Geometry check sheet. Reference: the model listing, model coordinates, mm. A direction names the side the tool comes from. Give positions to 0.01 mm unless a question says otherwise; leave off trailing zeros. Write each loop counter-clockwise with the first axis right and the second up, starting at its lowest first coordinate (ties: lowest second). Pieces come first, ordered by that corner, then holes. Notation, with made-up numbers: (-35, 31) -> (-6, 31) arc R22 cw to (-6, 60) -> close; hole circle Ø4 at (-1, 80). An arc over 180 degrees is marked (long way). One line per item, written item: value.
from build123d import *

# Parameters (mm, degrees)
V10_SHT_CANDIDATE_CARRIER16X16_START   = 54
SKETCH_2_W                             = 16
SKETCH_2_H                             = 1.6
V10_SHT_CANDIDATE_CARRIER16X16_DEPTH   = 16
V10_SHT_SENSING_PACKAGE_REARWARD_START = 60.5
SKETCH_3_W                             = 3
SKETCH_3_H                             = 1.2
V10_SHT_SENSING_PACKAGE_REARWARD_DEPTH = 3
SKETCH_4_R                             = 1.3
V10_SHT_TWO_CANDIDATE_HOLES8MM_DEPTH   = 1.6


with BuildPart() as part:
    # Sketch 2 → V10_SHT_candidate_carrier16x16 (new body)
    with BuildSketch(Plane.XY.offset(V10_SHT_CANDIDATE_CARRIER16X16_START)):
        with Locations((-122, 133.2)):
            Rectangle(SKETCH_2_W, SKETCH_2_H)
    extrude(amount=V10_SHT_CANDIDATE_CARRIER16X16_DEPTH)

    # Sketch 3 → V10_SHT_sensing_package_rearward (add)
    with BuildSketch(Plane.XY.offset(V10_SHT_SENSING_PACKAGE_REARWARD_START)):
        with Locations((-122, 134.6)):
            Rectangle(SKETCH_3_W, SKETCH_3_H)
    extrude(amount=V10_SHT_SENSING_PACKAGE_REARWARD_DEPTH)

    # Sketch 4 → V10_SHT_two_candidate_holes8mm (cut)
    with BuildSketch(Plane.XZ.offset(-132.4)):
        with Locations(Location((-126, 68, 0), (0, 0, 270))):
            Circle(SKETCH_4_R)
        with Locations(Location((-118, 68, 0), (0, 0, 270))):
            Circle(SKETCH_4_R)
    extrude(amount=-V10_SHT_TWO_CANDIDATE_HOLES8MM_DEPTH, mode=Mode.SUBTRACT)


solid = part.part
1) Depth check by flat-ended pin: pin 1 Ø1.3 at (x, y) = (-121.5, 135) entering from -Z; pin 2 Ø6 at (x, z) = (-123.5, 67) entering from +Y; pin 3 Ø1 at (y, z) = (135, 62) entering from -X. Enter the tip coordinate at first touch or a pass-through.
Verdict:
pin 1: z = 60.5
pin 2: y = 134
pin 3: x = -123.5
2) Sectioned sample at B-B on z = 68. Record the cut outline in (x, y).
Verdict:
outline: (-130, 132.4) -> (-127.3, 132.4) -> (-127.3, 134) -> (-130, 134) -> close; (-124.7, 132.4) -> (-119.3, 132.4) -> (-119.3, 134) -> (-124.7, 134) -> close; (-116.7, 132.4) -> (-114, 132.4) -> (-114, 134) -> (-116.7, 134) -> close
3) Mould release check, pull along Z, two halves, no side actions. Record for faces 4 (the flat face through (-122, 135, 60.5)), 5 (the flat face through (-122, 133, 70)), 6 (the flat face through (-123.5, 135, 62)), 7 (the cylindrical face through (-124.904, 133.189, 67.301)): released by +Z, released by -Z, zero draft, split by the parting line, or undercut.
Verdict:
face 4: released by -Z
face 5: released by +Z
face 6: zero draft
face 7: undercut
4) Sectioned sample at A-A on x = -126. Record the cut outline in (y, z), plus the area to 3 significant figures.
Verdict:
outline: (132.4, 54) -> (134, 54) -> (134, 66.7) -> (132.4, 66.7) -> close; (132.4, 69.3) -> (134, 69.3) -> (134, 70) -> (132.4, 70) -> close
area: 21.4 mm^2
5) Tool access check on faces 1 (the flat face through (-130, 133, 62)), 2 (the flat face through (-122, 135, 63.5)), 3 (the flat face through (-120.5, 135, 62)). Record the directions out of +Z, -Z, +X, -X, +Y, -Y that give a thin tool (end or side, any length) a straight path to the whole face; none if there is none.
Verdict:
face 1: +Z, -Z, -X, +Y, -Y
face 2: +Z, +X, -X, +Y
face 3: +Z, -Z, +X, +Y
6) Sectioned sample at C-C on y = 133.05. Record the cut outline in (x, z), plus the area to 3 significant figures.
Verdict:
outline: (-130, 54) -> (-114, 54) -> (-114, 70) -> (-130, 70) -> close; hole circle Ø2.6 at (-126, 68); hole circle Ø2.6 at (-118, 68)
area: 245 mm^2
7) Sectioned sample at D-D on z = 60.75. Record the cut outline in (x, y).
Verdict:
outline: (-130, 132.4) -> (-114, 132.4) -> (-114, 134) -> (-120.5, 134) -> (-120.5, 135.2) -> (-123.5, 135.2) -> (-123.5, 134) -> (-130, 134) -> close
8) Scan lines: probe 1 along X at (y, z) = (133.3, 68); probe 2 along X at (y, z) = (132.75, 67.5); probe 3 along Y at (x, z) = (-120.25, 62.75). Record each from-to range of solid material in increasing order.
Verdict:
probe 1: -130 to -127.3, -124.7 to -119.3, -116.7 to -114
probe 2: -130 to -127.2, -124.8 to -119.2, -116.8 to -114
probe 3: 132.4 to 134
